The drawing under review shows one solid part. Ordinate dimensions are in mm from its lowest x, y, z. Coordinates: 2 decimals unless noted, no trailing zeros. Order: outer loops, then holes, each group sorted by start corner. A loop starts at its lowest first (then second) coordinate and runs counter-clockwise, first axis right, second up.
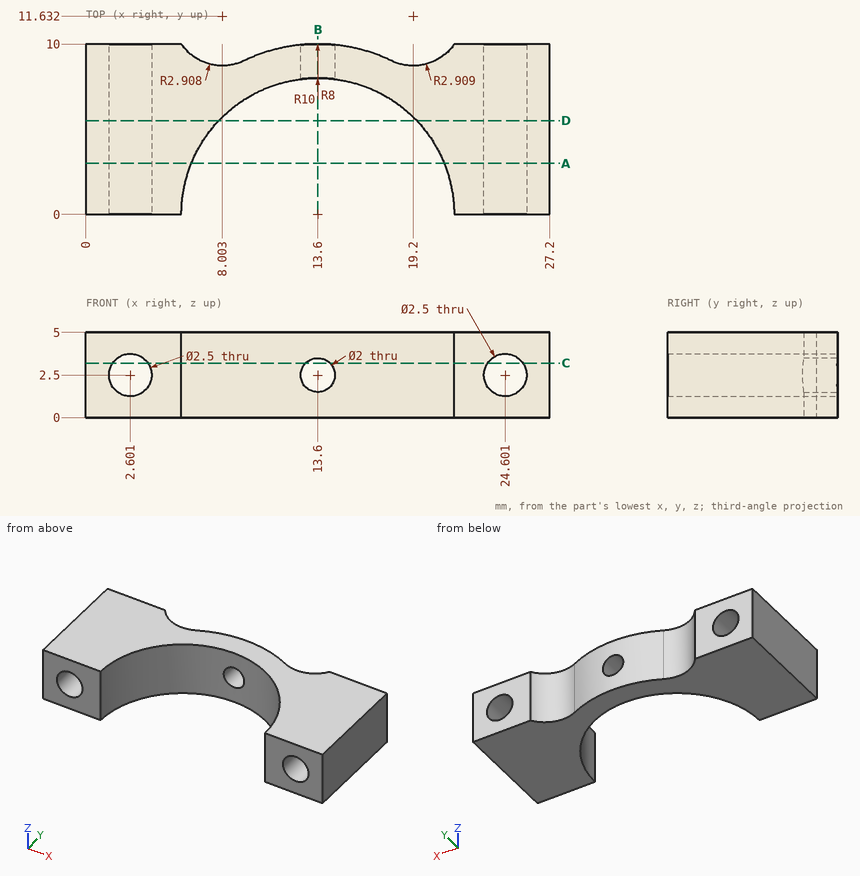
1. Take a section at A-A, the plane y = 3. Give the boundary of the cut face in (x, z).
Answer below:
outline: (0, 0) - (6.18, 0) - (6.18, 5) - (0, 5) - close; (21.02, 0) - (27.2, 0) - (27.2, 5) - (21.02, 5) - close; hole circle Ø2.5 at (2.6, 2.5); hole circle Ø2.5 at (24.6, 2.5)
2. Take a section at B-B, the plane x = 13.6. Give the boundary of the cut face in (y, z).
Answer below:
outline: (8, 0) - (10, 0) - (10, 1.5) - (8, 1.5) - close; (8, 3.5) - (10, 3.5) - (10, 5) - (8, 5) - close
3. Clearance check with a flat-ended pin moving along its axis: pin 1 Ø2 at (x, z) = (24.6, 2.5) entering from -Y. State where the tip first meets the part, or that it passes through.
Answer below:
pin 1: passes through
4. Take a section at D-D, the plane y = 5.5. Give the boundary of the cut face in (x, z).
Answer below:
outline: (0, 0) - (7.79, 0) - (7.79, 5) - (0, 5) - close; (19.41, 0) - (27.2, 0) - (27.2, 5) - (19.41, 5) - close; hole circle Ø2.5 at (2.6, 2.5); hole circle Ø2.5 at (24.6, 2.5)
5. To check wall thickness, follow L1, parallel to X at y = 5.5, z = 2.3 (1 decimal); L2, parallel to Z at x = 13.6, y = 9.6; L3, parallel to X at y = 4.25, z = 1.95 (1 decimal). State the ranges of each line that lie inside material, in increasing order.
Answer below:
L1: x = 0 to 1.4, 3.8 to 7.8, 19.4 to 23.4, 25.8 to 27.2
L2: z = 0 to 1.5, 3.5 to 5
L3: x = 0 to 1.5, 3.7 to 6.8, 20.4 to 23.5, 25.7 to 27.2
6. Take a section at C-C, the plane z = 3.2. Give the boundary of the cut face in (x, y) (1 decimal).
Answer below:
outline: (0, 0) - (1.6, 0) - (1.6, 10) - (0, 10) - close; (3.6, 0) - (5.6, 0) arc R8 cw to (12.9, 8) - (12.9, 10) arc R10 ccw to (9.3, 9) arc R2.9 cw to (5.6, 10) - (3.6, 10) - close; (14.3, 8) arc R8 cw to (21.6, 0) - (23.6, 0) - (23.6, 10) - (21.6, 10) arc R2.9 cw to (17.9, 9) arc R10 ccw to (14.3, 10) - close; (25.6, 0) - (27.2, 0) - (27.2, 10) - (25.6, 10) - close
